Verification items for the finished model (mm, model axes). Face numbers are marked on the shaded views. A direction names the side the tool comes from. Coordinates: 2 decimals unless noted, no trailing zeros. Loops run counter-clockwise (first coordinate to the right, second up) from the corner with the lowest first, then second, coordinate; pieces in that order, holes last. Notation, with made-up numbers: (71, -5.75) - (91, -5.75) arc R30 ccw to (91, 33.25) - close; hole circle Ø4 at (54.25, 81). An arc over 180 degrees is marked (long way). One line per item, written item: value. Start each with the question number.
(1) Gauge pin test, flat ends, axial feed: P1, Ø10, axis at x = -9.5, z = -10, coming from the +Y side; P2, Ø3, axis at x = -24.04, z = -24.04, coming from the +Y side; P3, Ø10, axis at y = 16, z = 21.5, coming from the -X side; P4, Ø5, axis at y = 12.5, z = 15, coming from the -X side. Record the tip position at first contact, or that the pin passes through.
(2) Section check C-C (z = -16). Record the boundary of the cut face in (x, y), plus the area to 3 significant figures.
(3) Set-up check for the marked faces 1 and 2: record each of +Z, -Z, +X, -X, +Y, -Y from which the full face is reachable in a straight line by a thin tool's end or side.
(4) Draft check along X on the marked faces 3, 4 and 5. Enter one of: +X half, -X half, draft (parallel to the pull), parting line (faces both ways), or undercut.
(5) Section check B-B (x = 0). Record the boundary of the cut face in (y, z).
(6) Thickness scan on probe 1 along Z at (x, y) = (25, 15); probe 2 along X at (y, z) = (10.25, 24). Record the ranges inside material, lowest first. Write a range as [from, to].
(7) Section check A-A (z = 0). Record the boundary of the cut face in (x, y), plus the area to 3 significant figures.
(8) Section check D-D (x = -8). Record the boundary of the cut face in (y, z), plus the area to 3 significant figures.
```python
from build123d import *

# Parameters (mm, degrees)
SKETCH1_R                = 33
BOSS_EXTRUDE1_DEPTH      = 4
SKETCH2_R                = 33
SKETCH2_R_2              = 31
BOSS_EXTRUDE2_DEPTH      = 16.88
M2_CLEARANCE_HOLE1_D     = 2.4
SKETCH13_R               = 2.5
CUT_EXTRUDE3_DEPTH       = 5
CUT_EXTRUDE2_DEPTH       = 5
SKETCH15_R               = 3
BOSS_EXTRUDE3_DEPTH      = 20.88
FILLET1_R                = 5
CIRPATTERN1_COUNT        = 4
FILLET1_OF_CIRPATTERN1_R = 5
F_3_0_MM_DOWEL_HOLES1_D  = 3.5


with BuildPart() as part:
    # Sketch1 → Boss-Extrude1 (new body)
    with BuildSketch(Plane(origin=(0, 0, 0), x_dir=(1, 0, 0), z_dir=(0, 1, 0))):
        Circle(SKETCH1_R)
    extrude(amount=BOSS_EXTRUDE1_DEPTH)

    # Sketch2 → Boss-Extrude2 (add)
    with BuildSketch(Plane(origin=(0, 4, 0), x_dir=(1, 0, 0), z_dir=(0, 1, 0))):
        Circle(SKETCH2_R)
        Circle(SKETCH2_R_2, mode=Mode.SUBTRACT)
    extrude(amount=BOSS_EXTRUDE2_DEPTH)

    # M2 Clearance Hole1 (through all)
    with Locations(Plane(origin=(0, 0, 0), x_dir=(-1, 0, 0), z_dir=(0, -1, 0))):
        with Locations((3.181980515, 3.181980515), (3.181980515, -3.181980515), (-3.181980515, -3.181980515), (-3.181980515, 3.181980515)):
            Hole(M2_CLEARANCE_HOLE1_D / 2)

    # Sketch13 → Cut-Extrude3 (cut, through all)
    with BuildSketch(Plane(origin=(0, 4, 0), x_dir=(1, 0, 0), z_dir=(0, 1, 0))):
        Circle(SKETCH13_R)
    extrude(amount=-CUT_EXTRUDE3_DEPTH, mode=Mode.SUBTRACT)

    # Sketch10 → Cut-Extrude2 (cut, through all)
    with BuildSketch(Plane(origin=(0, 4, 0), x_dir=(1, 0, 0), z_dir=(0, 1, 0))):
        with BuildLine():
            Line((13.5, -4), (13.5, 4))
            ThreePointArc((13.5, 4), (15, 5.5), (16.5, 4))
            Line((16.5, 4), (16.5, -4))
            ThreePointArc((16.5, -4), (15, -5.5), (13.5, -4))
        make_face()
    extrude(amount=-CUT_EXTRUDE2_DEPTH, mode=Mode.SUBTRACT)

    # Sketch15 → Boss-Extrude3 (add, through all)
    with BuildSketch(Plane(origin=(0, 20.88, 0), x_dir=(1, 0, 0), z_dir=(0, 1, 0))):
        with Locations((24.04163056, 24.04163056)):
            Circle(SKETCH15_R)
    boss_extrude3 = extrude(amount=-BOSS_EXTRUDE3_DEPTH)

    # Fillet1
    fillet1_edges = [part.edges().sort_by_distance(p)[0] for p in [
        (25.219946573, 10.44, -21.282722919),
        (21.282722919, 10.44, -25.219946573),
    ]]
    fillet(fillet1_edges, radius=FILLET1_R)

    # CirPattern1: Boss-Extrude3 ×4 about axis
    cirpattern1_axis = Axis((0, 0, 0), (0, 1, 0))
    for i in range(1, CIRPATTERN1_COUNT):
        add(boss_extrude3.rotate(cirpattern1_axis, i * 360 / CIRPATTERN1_COUNT))

    # Fillet1 of CirPattern1
    fillet1_of_cirpattern1_edges = [part.edges().sort_by_distance(p)[0] for p in [
        (-21.282722919, 10.44, -25.219946573),
        (-25.219946573, 10.44, -21.282722919),
        (-25.219946573, 10.44, 21.282722919),
        (-21.282722919, 10.44, 25.219946573),
        (21.282722919, 10.44, 25.219946573),
        (25.219946573, 10.44, 21.282722919),
    ]]
    fillet(fillet1_of_cirpattern1_edges, radius=FILLET1_OF_CIRPATTERN1_R)

    # Ø3.0 mm Dowel Holes1 (through all)
    with Locations(Plane(origin=(0, 20.88, 0), x_dir=(1, 0, 0), z_dir=(0, 1, 0))):
        with Locations((24.04163056, -24.04163056), (-24.04163056, -24.04163056), (-24.04163056, 24.04163056), (24.04163056, 24.04163056)):
            Hole(F_3_0_MM_DOWEL_HOLES1_D / 2)


solid = part.part
```
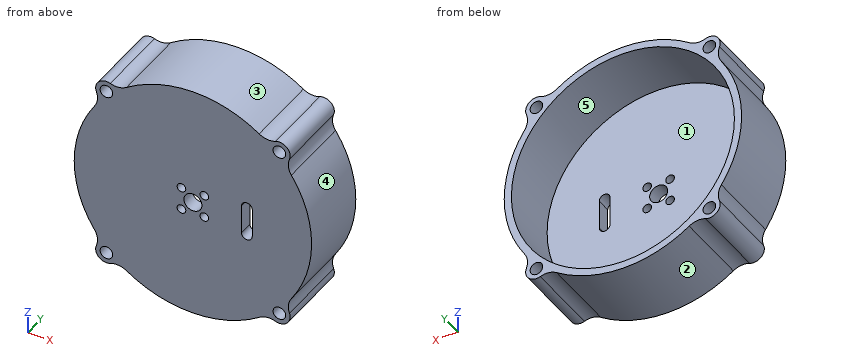
Responses:
1. P1: stops at y = 4
1. P2: passes through
1. P3: stops at x = -28.58
1. P4: stops at x = -30.54
2. outline: (-28.86, 0) - (28.86, 0) - (28.86, 20.88) - (26.55, 20.88) - (26.55, 4) - (-26.55, 4) - (-26.55, 20.88) - (-28.86, 20.88) - close
2. area: 309 mm²
3. face 1: +Y
3. face 2: -Z, +Y, -Y
4. face 3: parting line
4. face 4: +X half
4. face 5: undercut
5. outline: (0, -33) - (20.88, -33) - (20.88, -31) - (4, -31) - (4, -2.5) - (0, -2.5) - close; (0, 2.5) - (4, 2.5) - (4, 31) - (20.88, 31) - (20.88, 33) - (0, 33) - close
6. probe 1: z = [-26.88, -25.51], [-22.58, -18.33], [18.33, 22.58], [25.51, 26.88]
6. probe 2: x = [-27.04, -25.79], [-22.29, -19.62], [19.62, 22.29], [25.79, 27.04]
7. outline: (-33, 0) - (-2.5, 0) - (-2.5, 4) - (-31, 4) - (-31, 20.88) - (-33, 20.88) - close; (2.5, 0) - (13.5, 0) - (13.5, 4) - (2.5, 4) - close; (16.5, 0) - (33, 0) - (33, 20.88) - (31, 20.88) - (31, 4) - (16.5, 4) - close
7. area: 300 mm²
8. outline: (0, -32.02) - (20.88, -32.02) - (20.88, -29.95) - (4, -29.95) - (4, 29.95) - (20.88, 29.95) - (20.88, 32.02) - (0, 32.02) - close
8. area: 326 mm²
